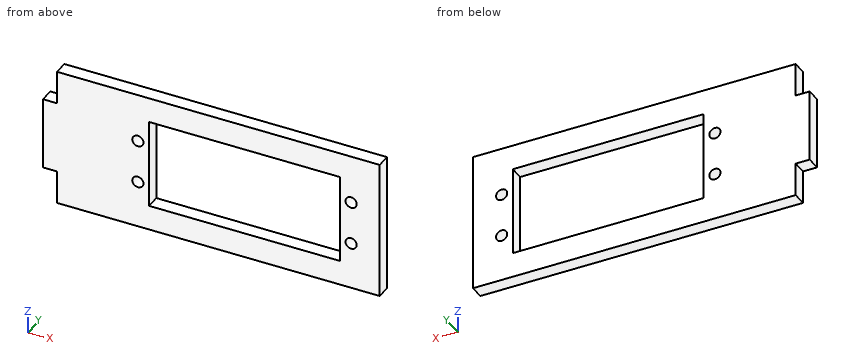
from build123d import *

# Parameters (mm, degrees)
SKETCH1_W           = 76.2
SKETCH1_H           = 31.75
BOSS_EXTRUDE1_DEPTH = 3.175
SKETCH2_R           = 1.27
SKETCH2_W           = 3.175
SKETCH2_H           = 7.62
SKETCH2_W_2         = 43.18
SKETCH2_H_2         = 20.32
CUT_EXTRUDE1_DEPTH  = 3.175


with BuildPart() as part:
    # Sketch1 → Boss-Extrude1 (new body)
    with BuildSketch(Plane(origin=(0, 0, 0), x_dir=(1, 0, 0), z_dir=(0, 1, 0))):
        with Locations((5.405536898, 2.364922393)):
            Rectangle(SKETCH1_W, SKETCH1_H)
    extrude(amount=BOSS_EXTRUDE1_DEPTH)

    # Sketch2 → Cut-Extrude1 (cut)
    with BuildSketch(Plane(origin=(0, 3.175, 0), x_dir=(1, 0, 0), z_dir=(0, 1, 0))):
        with Locations(Location((37.027343522, 7.508422393, 0), (0, 0, 270))):
            Circle(SKETCH2_R)
        with Locations(Location((37.027343522, -2.397577607, 0), (0, 0, 270))):
            Circle(SKETCH2_R)
        with Locations(Location((-11.232656478, 7.508422393, 0), (0, 0, 270))):
            Circle(SKETCH2_R)
        with Locations(Location((-11.232656478, -2.397577607, 0), (0, 0, 270))):
            Circle(SKETCH2_R)
        with Locations((-31.106963102, 14.429922393)):
            Rectangle(SKETCH2_W, SKETCH2_H)
        with Locations((-31.106963102, -9.700077607)):
            Rectangle(SKETCH2_W, SKETCH2_H)
        with Locations((12.897343522, 2.364922393)):
            Rectangle(SKETCH2_W_2, SKETCH2_H_2)
    extrude(amount=-CUT_EXTRUDE1_DEPTH, mode=Mode.SUBTRACT)


solid = part.part
Source: CAD feature listing. Evaluate the final solid. Frame: model axes, mm. Give positions to 0.01 mm unless a question says otherwise; leave off trailing zeros. Write each loop counter-clockwise with the first axis right and the second up, starting at its lowest first coordinate (ties: lowest second). Pieces come first, ordered by that corner, then holes. Notation, with made-up numbers: M -19,-13 L 27,-13 A12 ccw 27,10 Z; hole C 38.5,-27.75 d1. An arc over 180 degrees is marked long. Return JSON: item names as keys, results as strings. Group by question number.
1) Cut plane A-A, the plane x = -1.5. Output: boundary loops of the cut face in (y, z) (3 decimals), plus the area to 3 significant figures.
2) Cut plane D-D, the plane y = 1.05. Output: boundary loops of the cut face in (x, z), plus the area to 3 significant figures.
3) Cut plane C-C, the plane z = 3. Output: boundary loops of the cut face in (x, y) (3 decimals).
4) Material intervals for line 1 along Z through (x, y) = (37, 1.25); line 2 along Z through (x, y) = (18, 0.45); line 3 along X through (y, z) = (0.9, -12), sorted ascending. Write a range as [from, to].
5) Pin query (flat end, axial travel): P1, Ø1.5, axis at x = -11.23, z = 2.4, coming from the +Y side; P2, Ø1.6, axis at y = 2, z = -13.5, coming from the -X side; P3, Ø1.6, axis at x = -31.5, y = 1.5, coming from the +Z side. Return the tip coordinate at first contact, or that it passes through.
6) Cut plane B-B, the plane z = -0.5. Output: boundary loops of the cut face in (x, y) (3 decimals), plus the area to 3 significant figures.
Recorded:
{
 "1": {"outline": "M 0,-18.24 L 3.175,-18.24 L 3.175,-12.525 L 0,-12.525 Z; M 0,7.795 L 3.175,7.795 L 3.175,13.51 L 0,13.51 Z", "area": "36.3 mm²"},
 "2": {"outline": "M -32.69,-10.62 L -29.52,-10.62 L -29.52,-18.24 L 43.51,-18.24 L 43.51,13.51 L -29.52,13.51 L -29.52,5.89 L -32.69,5.89 Z; hole C -11.23,-7.51 d2.54; hole C -11.23,2.4 d2.54; hole M -8.69,-12.52 L 34.49,-12.52 L 34.49,7.8 L -8.69,7.8 Z; hole C 37.03,-7.51 d2.54; hole C 37.03,2.4 d2.54", "area": "1,470 mm²"},
 "3": {"outline": "M -32.694,0 L -12.351,0 L -12.351,3.175 L -32.694,3.175 Z; M -10.115,0 L -8.693,0 L -8.693,3.175 L -10.115,3.175 Z; M 34.487,0 L 35.909,0 L 35.909,3.175 L 34.487,3.175 Z; M 38.145,0 L 43.506,0 L 43.506,3.175 L 38.145,3.175 Z"},
 "4": {"line 1": "z = [-18.24, -8.78], [-6.24, 1.13], [3.67, 13.51]", "line 2": "z = [-18.24, -12.52], [7.8, 13.51]", "line 3": "x = [-29.52, -8.69], [34.49, 43.51]"},
 "5": {"P1": "passes through", "P2": "stops at x = -29.52", "P3": "stops at z = 5.89"},
 "6": {"outline": "M -32.694,0 L -8.693,0 L -8.693,3.175 L -32.694,3.175 Z; M 34.487,0 L 43.506,0 L 43.506,3.175 L 34.487,3.175 Z", "area": "105 mm²"}
}
